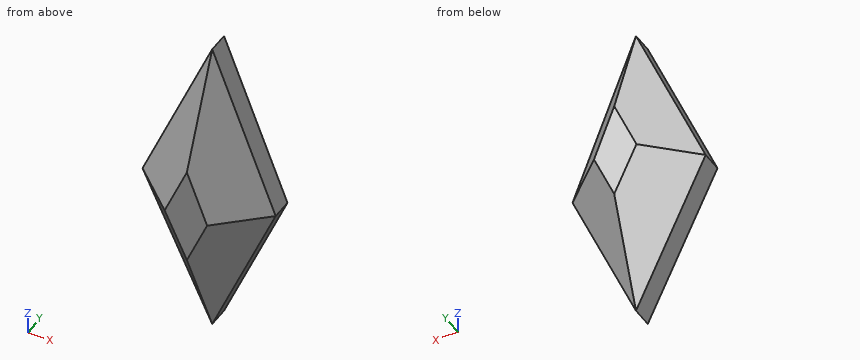
```python
from build123d import *

# Parameters (mm, degrees)
F1_DEPTH = 25
F2_SIZE  = 10


with BuildPart() as f1:
    # F0 (on Front) → F1 (new body)
    with BuildSketch(Plane.XZ):
        Polygon((0, 39.001424), (-16.736243, 0), (0, -35.415087), (15.241938, 0), align=None)
    extrude(amount=F1_DEPTH)

    # F2
    f2_edges = [f1.edges().sort_by_distance(p)[0] for p in [
        (-8.368121, -25, 19.500712),
        (-8.368121, 0, 19.500712),
        (-8.368121, -25, -17.707543),
        (-8.368121, 0, -17.707543),
        (7.620969, 0, 19.500712),
        (7.620969, -25, 19.500712),
        (7.620969, -25, -17.707543),
        (7.620969, 0, -17.707543),
    ]]
    chamfer(f2_edges, length=F2_SIZE)


solid = f1.part
```
Model file for the job. Use its own axes, mm. Round coordinates to 2 decimals unless told otherwise and drop trailing zeros. Order: outer loops, then holes, each group sorted by start corner. A loop starts at its lowest first (then second) coordinate and runs counter-clockwise, first axis right, second up. Notation, with made-up numbers: (48.25, -14) -> (56.25, -14) arc R26 cw to (56.25, 20) -> close; hole circle Ø4 at (42.5, 55). An arc over 180 degrees is marked (long way). Use one line per item in the form item = value.
Item 1: Flat gauge pins, fed straight in: pin 1 Ø3 at (x, z) = (-3, 19.5) entering from +Y; pin 2 Ø8 at (x, z) = (4, 20.5) entering from -Y; pin 3 Ø8 at (y, z) = (-15, 5) entering from +X. Where does each tip first touch, or does it go through?
Returned:
pin_1 = -3.57
pin_2 = -22.01
pin_3 = 14.85
Item 2: Cut at B-B, the plane x = -4.5. Write the cut outline in (y, z), and give its area (3 significant figures).
Returned:
outline = (-25, -2.49) -> (-15, -25.89) -> (-10, -25.89) -> (0, -2.49) -> (0, 3.16) -> (-10, 28.51) -> (-15, 28.51) -> (-25, 3.16) -> close
area = 873 mm^2
Item 3: Drill centre lines: line 1 (X direction, y = -6.5, z = -2.5); line 2 (X direction, y = -5.5, z = 21.5); line 3 (Y direction, x = 7.5, z = 19.5). Where is each one in solid material? Low to high.
Returned:
line_1 = -11.68 to 10.36
line_2 = -2.61 to 2.01
line_3 = -15.11 to -9.89
Item 4: Cut at A-A, the plane z = -10. Write the cut outline in (x, y), and give its area (3 significant figures).
Returned:
outline = (-12.01, -15) -> (-0.95, -25) -> (0.05, -25) -> (10.94, -15) -> (10.94, -10) -> (0.05, 0) -> (-0.95, 0) -> (-12.01, -10) -> close
area = 354 mm^2
Item 5: Cut at D-D, the plane z = -29.5. Write the cut outline in (x, y).
Returned:
outline = (-2.8, -15) -> (-0.1, -17.43) -> (2.55, -15) -> (2.55, -10) -> (-0.1, -7.57) -> (-2.8, -10) -> close
Item 6: Cut at C-C, the plane y = -10.75. Write the cut outline in (x, z), and give its area (3 significant figures).
Returned:
outline = (-16.74, 0) -> (0, -35.42) -> (15.24, 0) -> (0, 39) -> close
area = 1,190 mm^2
